Here's how the part is built. I have some questions about the finished solid (model axes, mm). Round coordinates to 2 decimals unless told otherwise and drop trailing zeros. Order: outer loops, then holes, each group sorted by start corner. A loop starts at its lowest first (then second) coordinate and runs counter-clockwise, first axis right, second up. Notation, with made-up numbers: (-17, -25.75) -> (-2, -25.75) arc R17 ccw to (-2, -14.75) -> close; hole circle Ø7 at (-6, -15). An arc over 180 degrees is marked (long way). Use a Markdown table: item, result. Add a question column.
(1) I want a section at A-A, the plane x = -5. Please give me the cut outline in (y, z).
(2) I want a section at C-C, the plane z = -83. Please give me the cut outline in (x, y).
(3) I'm going to push flat-ended pins straight in: P1, Ø9, axis at x = -15, z = -20, coming from the +Y side; P2, Ø9.5, axis at x = -105, z = -20, coming from the +Y side. Where does each tip first touch, or does it pass through?
(4) If I drill on probe 1 along X at (y, z) = (1.15, -20); probe 2 along X at (y, z) = (1.45, -53); probe 3 along Z at (x, y) = (-60, 0.6), over which ranges is the centre line in solid material (lowest first)?
(5) I want a section at B-B, the plane z = -5. Please give me the cut outline in (x, y), then the cut area to 3 significant figures.
(6) I want a section at D-D, the plane y = 1.65. Give the number of separate pieces and of enclosed holes in the cut face, then the cut area to 3 significant figures.
(7) Thinking about a two-plate mould opening in Z: for faces 1 (the face through (-48.65, 1.01, -57.76)), 2 (the face through (-70.94, 1.01, -57.42)), 3 (the face through (-61, 2, -51)), which applies, pulls with the +Z half, pulls with the -Z half, needs draft (parallel to the pull), parting line crosses it, or undercut?
from build123d import *

# Parameters (mm, degrees)
BOTTOM_PLATE_W                       = 120
BOTTOM_PLATE_H                       = 100
BOTTOM_PLATE_EXT_DEPTH               = 2
MIDDLE_ROW_R                         = 6
MIDDLE_ROW_CUT_DEPTH                 = 157.217796681
TOP_ROW_R                            = 8.25
TOP_ROW_R_2                          = 6.1
TOP_ROW_CUT_DEPTH                    = 157.217796681
BOTTOM_ROW_R                         = 3.55
BOTTOM_ROW_R_2                       = 6
BOTTOM_ROW_CUT_DEPTH                 = 157.217796681
PLATE_SCREWS_R                       = 1.65
PLATE_SCREWS_CUT_DEPTH               = 157.217796681
PLATE_SCREW_HEAD_R                   = 2.8
PLATE_SCREW_HEAD_CUT_DEPTH           = 2
PLATE_SCREW_HEAD_CUT_DRAFT           = -45
PLATE_SCREW_HEAD_CUT_PROFILE_2_DEPTH = 2
PLATE_SCREW_HEAD_CUT_PROFILE_2_DRAFT = -45
PLATE_SCREW_HEAD_CUT_PROFILE_3_DEPTH = 2
PLATE_SCREW_HEAD_CUT_PROFILE_3_DRAFT = -45
PLATE_SCREW_HEAD_CUT_PROFILE_4_DEPTH = 2
PLATE_SCREW_HEAD_CUT_PROFILE_4_DRAFT = -45
PLATE_SCREW_HEAD_CUT_PROFILE_5_DEPTH = 2
PLATE_SCREW_HEAD_CUT_PROFILE_5_DRAFT = -45
PLATE_SCREW_HEAD_CUT_PROFILE_6_DEPTH = 2
PLATE_SCREW_HEAD_CUT_PROFILE_6_DRAFT = -45
FILLET1_R                            = 2
FILLET2_R                            = 2
FILLET3_R                            = 2
FILLET4_R                            = 2


with BuildPart() as part:
    # Bottom Plate → Bottom Plate EXT (new body)
    with BuildSketch(Plane(origin=(0, 0, 0), x_dir=(1, 0, 0), z_dir=(0, 1, 0))):
        with Locations((-60, 50)):
            Rectangle(BOTTOM_PLATE_W, BOTTOM_PLATE_H)
    extrude(amount=BOTTOM_PLATE_EXT_DEPTH)

    # Middle Row → Middle Row Cut (cut, through all)
    with BuildSketch(Plane(origin=(0, 2, 0), x_dir=(1, 0, 0), z_dir=(0, 1, 0))):
        with Locations(Location((-105, 53, 0), (0, 0, 270))):
            Circle(MIDDLE_ROW_R)
        with Locations(Location((-75, 53, 0), (0, 0, 270))):
            Circle(MIDDLE_ROW_R)
        with Locations(Location((-45, 53, 0), (0, 0, 270))):
            Circle(MIDDLE_ROW_R)
        with Locations(Location((-15, 53, 0), (0, 0, 270))):
            Circle(MIDDLE_ROW_R)
    extrude(amount=-MIDDLE_ROW_CUT_DEPTH, mode=Mode.SUBTRACT)

    # Top Row → Top Row Cut (cut, through all)
    with BuildSketch(Plane(origin=(0, 2, 0), x_dir=(1, 0, 0), z_dir=(0, 1, 0))):
        with Locations(Location((-105, 83, 0), (0, 0, 270))):
            Circle(TOP_ROW_R)
        with Locations(Location((-75, 83, 0), (0, 0, 270))):
            Circle(TOP_ROW_R_2)
        with Locations(Location((-45, 83, 0), (0, 0, 270))):
            Circle(TOP_ROW_R_2)
        with Locations(Location((-15, 83, 0), (0, 0, 270))):
            Circle(TOP_ROW_R_2)
    extrude(amount=-TOP_ROW_CUT_DEPTH, mode=Mode.SUBTRACT)

    # Bottom Row → Bottom Row Cut (cut, through all)
    with BuildSketch(Plane(origin=(0, 2, 0), x_dir=(1, 0, 0), z_dir=(0, 1, 0))):
        with Locations(Location((-75, 20, 0), (0, 0, 270))):
            Circle(BOTTOM_ROW_R)
        with Locations(Location((-45, 20, 0), (0, 0, 270))):
            Circle(BOTTOM_ROW_R)
        with Locations(Location((-15, 20, 0), (0, 0, 270))):
            Circle(BOTTOM_ROW_R)
        with Locations(Location((-105, 20, 0), (0, 0, 270))):
            Circle(BOTTOM_ROW_R_2)
    extrude(amount=-BOTTOM_ROW_CUT_DEPTH, mode=Mode.SUBTRACT)

    # Plate Screws → Plate Screws Cut (cut, through all)
    with BuildSketch(Plane(origin=(0, 2, 0), x_dir=(1, 0, 0), z_dir=(0, 1, 0))):
        with Locations(Location((-115, 95, 0), (0, 0, 270))):
            Circle(PLATE_SCREWS_R)
        with Locations(Location((-5, 95, 0), (0, 0, 270))):
            Circle(PLATE_SCREWS_R)
        with Locations(Location((-5, 5, 0), (0, 0, 270))):
            Circle(PLATE_SCREWS_R)
        with Locations(Location((-115, 5, 0), (0, 0, 270))):
            Circle(PLATE_SCREWS_R)
        with Locations(Location((-60, 95, 0), (0, 0, 270))):
            Circle(PLATE_SCREWS_R)
        with Locations(Location((-60, 5, 0), (0, 0, 90))):
            Circle(PLATE_SCREWS_R)
    extrude(amount=-PLATE_SCREWS_CUT_DEPTH, mode=Mode.SUBTRACT)


with BuildPart() as plate_screw_head_cut_tool:
    # Plate Screw Head → Plate Screw Head Cut (with draft: the straight prism first)
    with BuildSketch(Plane(origin=(0, 2, 0), x_dir=(1, 0, 0), z_dir=(0, 1, 0))):
        with Locations((-115, 95)):
            Circle(PLATE_SCREW_HEAD_R)
    extrude(amount=-PLATE_SCREW_HEAD_CUT_DEPTH)
    # Plate Screw Head Cut: the draft: its side faces are tilted about the plane it starts from
    plate_screw_head_cut_sides = [plate_screw_head_cut_tool.faces().sort_by_distance(p)[0] for p in [
        (-117.8, 1, -95),
    ]]
    draft(plate_screw_head_cut_sides, Plane(origin=(0, 2, 0), x_dir=(1, 0, 0), z_dir=(0, 1, 0)), PLATE_SCREW_HEAD_CUT_DRAFT)


with BuildPart() as part_1:
    add(part.part)

    # Plate Screw Head Cut: cut by plate_screw_head_cut_tool
    add(plate_screw_head_cut_tool.part, mode=Mode.SUBTRACT)


with BuildPart() as plate_screw_head_cut_profile_2_tool:
    # Plate Screw Head → Plate Screw Head Cut profile 2 (with draft: the straight prism first)
    with BuildSketch(Plane(origin=(0, 2, 0), x_dir=(1, 0, 0), z_dir=(0, 1, 0))):
        with Locations((-5, 95)):
            Circle(PLATE_SCREW_HEAD_R)
    extrude(amount=-PLATE_SCREW_HEAD_CUT_PROFILE_2_DEPTH)
    # Plate Screw Head Cut profile 2: the draft: its side faces are tilted about the plane it starts from
    plate_screw_head_cut_profile_2_sides = [plate_screw_head_cut_profile_2_tool.faces().sort_by_distance(p)[0] for p in [
        (-7.8, 1, -95),
    ]]
    draft(plate_screw_head_cut_profile_2_sides, Plane(origin=(0, 2, 0), x_dir=(1, 0, 0), z_dir=(0, 1, 0)), PLATE_SCREW_HEAD_CUT_PROFILE_2_DRAFT)


with BuildPart() as part_2:
    add(part_1.part)

    # Plate Screw Head Cut profile 2: cut by plate_screw_head_cut_profile_2_tool
    add(plate_screw_head_cut_profile_2_tool.part, mode=Mode.SUBTRACT)


with BuildPart() as plate_screw_head_cut_profile_3_tool:
    # Plate Screw Head → Plate Screw Head Cut profile 3 (with draft: the straight prism first)
    with BuildSketch(Plane(origin=(0, 2, 0), x_dir=(1, 0, 0), z_dir=(0, 1, 0))):
        with Locations((-5, 5)):
            Circle(PLATE_SCREW_HEAD_R)
    extrude(amount=-PLATE_SCREW_HEAD_CUT_PROFILE_3_DEPTH)
    # Plate Screw Head Cut profile 3: the draft: its side faces are tilted about the plane it starts from
    plate_screw_head_cut_profile_3_sides = [plate_screw_head_cut_profile_3_tool.faces().sort_by_distance(p)[0] for p in [
        (-7.8, 1, -5),
    ]]
    draft(plate_screw_head_cut_profile_3_sides, Plane(origin=(0, 2, 0), x_dir=(1, 0, 0), z_dir=(0, 1, 0)), PLATE_SCREW_HEAD_CUT_PROFILE_3_DRAFT)


with BuildPart() as part_3:
    add(part_2.part)

    # Plate Screw Head Cut profile 3: cut by plate_screw_head_cut_profile_3_tool
    add(plate_screw_head_cut_profile_3_tool.part, mode=Mode.SUBTRACT)


with BuildPart() as plate_screw_head_cut_profile_4_tool:
    # Plate Screw Head → Plate Screw Head Cut profile 4 (with draft: the straight prism first)
    with BuildSketch(Plane(origin=(0, 2, 0), x_dir=(1, 0, 0), z_dir=(0, 1, 0))):
        with Locations((-115, 5)):
            Circle(PLATE_SCREW_HEAD_R)
    extrude(amount=-PLATE_SCREW_HEAD_CUT_PROFILE_4_DEPTH)
    # Plate Screw Head Cut profile 4: the draft: its side faces are tilted about the plane it starts from
    plate_screw_head_cut_profile_4_sides = [plate_screw_head_cut_profile_4_tool.faces().sort_by_distance(p)[0] for p in [
        (-117.8, 1, -5),
    ]]
    draft(plate_screw_head_cut_profile_4_sides, Plane(origin=(0, 2, 0), x_dir=(1, 0, 0), z_dir=(0, 1, 0)), PLATE_SCREW_HEAD_CUT_PROFILE_4_DRAFT)


with BuildPart() as part_4:
    add(part_3.part)

    # Plate Screw Head Cut profile 4: cut by plate_screw_head_cut_profile_4_tool
    add(plate_screw_head_cut_profile_4_tool.part, mode=Mode.SUBTRACT)


with BuildPart() as plate_screw_head_cut_profile_5_tool:
    # Plate Screw Head → Plate Screw Head Cut profile 5 (with draft: the straight prism first)
    with BuildSketch(Plane(origin=(0, 2, 0), x_dir=(1, 0, 0), z_dir=(0, 1, 0))):
        with Locations((-60, 95)):
            Circle(PLATE_SCREW_HEAD_R)
    extrude(amount=-PLATE_SCREW_HEAD_CUT_PROFILE_5_DEPTH)
    # Plate Screw Head Cut profile 5: the draft: its side faces are tilted about the plane it starts from
    plate_screw_head_cut_profile_5_sides = [plate_screw_head_cut_profile_5_tool.faces().sort_by_distance(p)[0] for p in [
        (-62.8, 1, -95),
    ]]
    draft(plate_screw_head_cut_profile_5_sides, Plane(origin=(0, 2, 0), x_dir=(1, 0, 0), z_dir=(0, 1, 0)), PLATE_SCREW_HEAD_CUT_PROFILE_5_DRAFT)


with BuildPart() as part_5:
    add(part_4.part)

    # Plate Screw Head Cut profile 5: cut by plate_screw_head_cut_profile_5_tool
    add(plate_screw_head_cut_profile_5_tool.part, mode=Mode.SUBTRACT)


with BuildPart() as plate_screw_head_cut_profile_6_tool:
    # Plate Screw Head → Plate Screw Head Cut profile 6 (with draft: the straight prism first)
    with BuildSketch(Plane(origin=(0, 2, 0), x_dir=(1, 0, 0), z_dir=(0, 1, 0))):
        with Locations((-60, 5)):
            Circle(PLATE_SCREW_HEAD_R)
    extrude(amount=-PLATE_SCREW_HEAD_CUT_PROFILE_6_DEPTH)
    # Plate Screw Head Cut profile 6: the draft: its side faces are tilted about the plane it starts from
    plate_screw_head_cut_profile_6_sides = [plate_screw_head_cut_profile_6_tool.faces().sort_by_distance(p)[0] for p in [
        (-62.8, 1, -5),
    ]]
    draft(plate_screw_head_cut_profile_6_sides, Plane(origin=(0, 2, 0), x_dir=(1, 0, 0), z_dir=(0, 1, 0)), PLATE_SCREW_HEAD_CUT_PROFILE_6_DRAFT)


with BuildPart() as part_6:
    add(part_5.part)

    # Plate Screw Head Cut profile 6: cut by plate_screw_head_cut_profile_6_tool
    add(plate_screw_head_cut_profile_6_tool.part, mode=Mode.SUBTRACT)

    # Fillet1
    fillet1_edges = [part_6.edges().sort_by_distance(p)[0] for p in [
        (-120, 1, -100),
    ]]
    fillet(fillet1_edges, radius=FILLET1_R)

    # Fillet2
    fillet2_edges = [part_6.edges().sort_by_distance(p)[0] for p in [
        (0, 1, -100),
    ]]
    fillet(fillet2_edges, radius=FILLET2_R)

    # Fillet3
    fillet3_edges = [part_6.edges().sort_by_distance(p)[0] for p in [
        (0, 1, 0),
    ]]
    fillet(fillet3_edges, radius=FILLET3_R)

    # Fillet4
    fillet4_edges = [part_6.edges().sort_by_distance(p)[0] for p in [
        (-120, 1, 0),
    ]]
    fillet(fillet4_edges, radius=FILLET4_R)


solid = part_6.part
Taken from the geometry:
| question | item | result |
|---|---|---|
| 1 | outline | (0, -100) -> (2, -100) -> (2, -97.8) -> (0.85, -96.65) -> (0, -96.65) -> close; (0, -93.35) -> (0.85, -93.35) -> (2, -92.2) -> (2, -7.8) -> (0.85, -6.65) -> (0, -6.65) -> close; (0, -3.35) -> (0.85, -3.35) -> (2, -2.2) -> (2, 0) -> (0, 0) -> close |
| 2 | outline | (-120, 0) -> (-113.25, 0) -> (-113.25, 2) -> (-120, 2) -> close; (-96.75, 0) -> (-81.1, 0) -> (-81.1, 2) -> (-96.75, 2) -> close; (-68.9, 0) -> (-51.1, 0) -> (-51.1, 2) -> (-68.9, 2) -> close; (-38.9, 0) -> (-21.1, 0) -> (-21.1, 2) -> (-38.9, 2) -> close; (-8.9, 0) -> (0, 0) -> (0, 2) -> (-8.9, 2) -> close |
| 3 | P1 | stops at y = 2 |
| 3 | P2 | passes through |
| 4 | probe 1 | x = -120 to -111, -99 to -78.55, -71.45 to -48.55, -41.45 to -18.55, -11.45 to 0 |
| 4 | probe 2 | x = -120 to -111, -99 to -81, -69 to -51, -39 to -21, -9 to 0 |
| 4 | probe 3 | z = -100 to -96.65, -93.35 to -6.65, -3.35 to 0 |
| 5 | outline | (-120, 0) -> (-116.65, 0) -> (-116.65, 0.85) -> (-117.8, 2) -> (-120, 2) -> close; (-113.35, 0) -> (-61.65, 0) -> (-61.65, 0.85) -> (-62.8, 2) -> (-112.2, 2) -> (-113.35, 0.85) -> close; (-58.35, 0) -> (-6.65, 0) -> (-6.65, 0.85) -> (-7.8, 2) -> (-57.2, 2) -> (-58.35, 0.85) -> close; (-3.35, 0) -> (0, 0) -> (0, 2) -> (-2.2, 2) -> (-3.35, 0.85) -> close |
| 5 | area | 216 mm2 |
| 6 | separate pieces | 1 |
| 6 | enclosed holes | 18 |
| 6 | area | 10,600 mm2 |
| 7 | face 1 | undercut |
| 7 | face 2 | undercut |
| 7 | face 3 | needs draft |
